Input: part model. Units: mm. Frame: model coordinates. Face numbers are marked on the shaded views. A direction names the side the tool comes from. Round coordinates to 2 decimals unless told otherwise and drop trailing zeros. Order: outer loops, then holes, each group sorted by start corner. A loop starts at its lowest first (then second) coordinate and runs counter-clockwise, first axis right, second up. Notation, with made-up numbers: (71.25, 46.5) -> (85.25, 46.5) arc R18 ccw to (85.25, 81.5) -> close; hole circle Ø1 at (-20.5, 44). An arc over 180 degrees is marked (long way). Answer as CSV lines item,"result". Start each with the question number.
1) Line query: L1, parallel to Y at x = 55, z = -3; L2, parallel to Y at x = 14, z = -6.8; L3, parallel to Y at x = 14, z = -2. Output: solid intervals per line, ascending.
2) Section query B-B, the plane z = -24. Output: boundary loops of the cut face in (x, y).
3) Section query A-A, the plane y = -102. Output: boundary loops of the cut face in (x, z), and give its area (3 significant figures).
4) Section query D-D, the plane y = -25. Output: boundary loops of the cut face in (x, z).
5) Section query C-C, the plane y = -78. Output: boundary loops of the cut face in (x, z), and give its area (3 significant figures).
6) Access query for the marked faces 1, 2 and 3. Directions: +Z, -Z, +X, -X, +Y, -Y. A direction counts if a zero-diameter tool reaches every point of the face in a straight line with its end or side. Return the directions, or none.
7) First-contact query: P1, Ø9, axis at x = 14, y = -15, coming from the +Z side; P2, Ø5, axis at x = 14, y = -15, coming from the +Z side; P3, Ø8, axis at x = 112, z = -22, coming from the +Y side; P4, Ø8, axis at x = 171.5, y = -84.5, coming from the +Z side. Flat tips, straight axial feed; report the tip coordinate or a pass-through.
```python
from build123d import *

# Parameters (mm, degrees)
SKETCH2_W           = 230
SKETCH2_H           = 120
BOSS_EXTRUDE1_DEPTH = 38
CUT_EXTRUDE1_DEPTH  = 28
SKETCH4_W           = 160
SKETCH4_H           = 46
CUT_EXTRUDE2_DEPTH  = 261.929109147
SKETCH5_R           = 3
CUT_EXTRUDE3_DEPTH  = 10
SKETCH9_W           = 276.739384021
SKETCH9_H           = 54.976414544
CUT_EXTRUDE5_DEPTH  = 263.190770242
SKETCH6_R           = 3
CUT_EXTRUDE4_DEPTH  = 260.563094449
SKETCH10_R          = 5
CUT_EXTRUDE6_DEPTH  = 6
SKETCH11_R          = 2
CUT_EXTRUDE7_DEPTH  = 261.831363145
SKETCH12_R          = 2.5
CUT_EXTRUDE8_DEPTH  = 261.831363145


with BuildPart() as part:
    # Sketch2 → Boss-Extrude1 (new body)
    with BuildSketch(Plane.XY):
        with Locations((115, -60)):
            Rectangle(SKETCH2_W, SKETCH2_H)
    extrude(amount=BOSS_EXTRUDE1_DEPTH)

    # Sketch3 → Cut-Extrude1 (cut)
    with BuildSketch(Plane.XY.offset(38)):
        Polygon((28, -120), (28, -74), (230, -74), (230, 0), (0, 0), (0, -120), align=None)
    extrude(amount=-CUT_EXTRUDE1_DEPTH, mode=Mode.SUBTRACT)

    # Sketch4 → Cut-Extrude2 (cut, through all)
    with BuildSketch(Plane.XY.offset(10)):
        with Locations((150, -23)):
            Rectangle(SKETCH4_W, SKETCH4_H)
    extrude(amount=-CUT_EXTRUDE2_DEPTH, mode=Mode.SUBTRACT)


with BuildPart() as body_2:
    # Mirror2: mirrored copy
    add(part.part.mirror(Plane(origin=(102.272727273, -73.454545455, 0), x_dir=(1, 0, 0), z_dir=(0, 0, -1))))

    # Sketch5 → Cut-Extrude3 (cut)
    with BuildSketch(Plane(origin=(0, -74, 0), x_dir=(1, 0, 0), z_dir=(0, 1, 0))):
        with Locations(Location((128, 24, 0), (0, 0, 270))):
            Circle(SKETCH5_R)
    extrude(amount=-CUT_EXTRUDE3_DEPTH, mode=Mode.SUBTRACT)

    # Sketch9 → Cut-Extrude5 (cut, through all)
    with BuildSketch(Plane(origin=(0, 0, -38), x_dir=(-1, 0, 0), z_dir=(0, 0, -1))):
        with Locations((-118.343160344, -144.488207272)):
            Rectangle(SKETCH9_W, SKETCH9_H)
    extrude(amount=-CUT_EXTRUDE5_DEPTH, mode=Mode.SUBTRACT)

    # Sketch6 → Cut-Extrude4 (cut, through all)
    with BuildSketch(Plane(origin=(0, 0, -10), x_dir=(-1, 0, 0), z_dir=(0, 0, -1))):
        with Locations((-14, -102)):
            Circle(SKETCH6_R)
        with Locations((-14, -15)):
            Circle(SKETCH6_R)
    extrude(amount=-CUT_EXTRUDE4_DEPTH, mode=Mode.SUBTRACT)

    # Sketch10 → Cut-Extrude6 (cut)
    with BuildSketch(Plane.XY):
        with Locations((14, -15)):
            Circle(SKETCH10_R)
        with Locations((14, -102)):
            Circle(SKETCH10_R)
    extrude(amount=-CUT_EXTRUDE6_DEPTH, mode=Mode.SUBTRACT)

    # Sketch11 → Cut-Extrude7 (cut, through all)
    with BuildSketch(Plane.XY):
        with Locations((55, -40)):
            Circle(SKETCH11_R)
        with Locations((55, -10)):
            Circle(SKETCH11_R)
        with Locations((32, -10)):
            Circle(SKETCH11_R)
        with Locations((32, -40)):
            Circle(SKETCH11_R)
    extrude(amount=-CUT_EXTRUDE7_DEPTH, mode=Mode.SUBTRACT)

    # Sketch12 → Cut-Extrude8 (cut, through all)
    with BuildSketch(Plane.XY):
        with Locations((16, -25)):
            Circle(SKETCH12_R)
    extrude(amount=-CUT_EXTRUDE8_DEPTH, mode=Mode.SUBTRACT)


solid = body_2.part
```
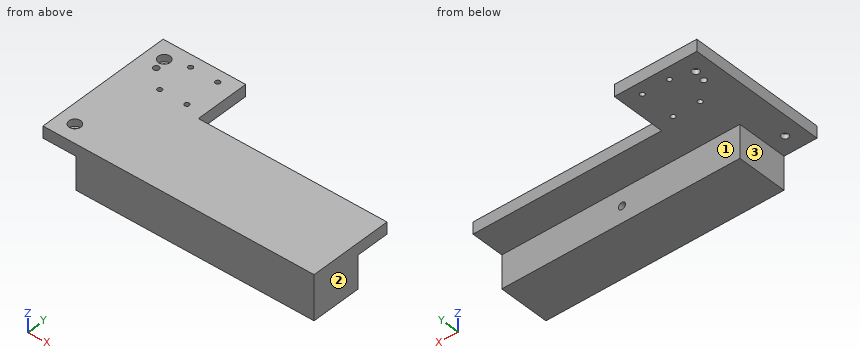
Findings:
1,L1,"y = -117 to -42, -38 to -12, -8 to 0"
1,L2,"y = -117 to -105, -99 to -26.5, -23.5 to -18, -12 to 0"
1,L3,"y = -117 to -107, -97 to -26.5, -23.5 to -20, -10 to 0"
2,outline,"(28, -117) -> (230, -117) -> (230, -74) -> (131, -74) -> (131, -84) -> (125, -84) -> (125, -74) -> (28, -74) -> close"
3,outline,"(0, -10) -> (11, -10) -> (11, -6) -> (9, -6) -> (9, 0) -> (0, 0) -> close; (17, -10) -> (28, -10) -> (28, -38) -> (230, -38) -> (230, 0) -> (19, 0) -> (19, -6) -> (17, -6) -> close"
3,area,"7,870 mm^2"
4,outline,"(0, -10) -> (13.5, -10) -> (13.5, 0) -> (0, 0) -> close; (18.5, -10) -> (70, -10) -> (70, 0) -> (18.5, 0) -> close"
5,outline,"(0, -10) -> (28, -10) -> (28, -38) -> (230, -38) -> (230, 0) -> (0, 0) -> close; hole circle Ø6 at (128, -24)"
5,area,"7,930 mm^2"
6,face 1,"-Z, +X, -X, +Y"
6,face 2,"+Z, -Z, +X, +Y, -Y"
6,face 3,"-Z, -X, +Y, -Y"
7,P1,"stops at z = -6"
7,P2,"passes through"
7,P3,"stops at y = -74"
7,P4,"stops at z = 0"
